```python
from build123d import *

# Parameters (mm, degrees)
BOSS_EXTRUDE1_DEPTH = 36.5
CUT_EXTRUDE1_DEPTH  = 119.232821162
SKETCH3_W           = 12
SKETCH3_H           = 22
CUT_EXTRUDE4_DEPTH  = 7
SKETCH7_R           = 1.5
CUT_EXTRUDE10_DEPTH = 8


with BuildPart() as part:
    # Sketch1 → Boss-Extrude1 (new, symmetric)
    with BuildSketch(Plane.XY):
        Polygon((-55, 0), (55, 0), (55, 15), (29.503066419, 15), (20, 75), (-20, 75), (-29.503066419, 15), (-55, 15), align=None)
    extrude(amount=BOSS_EXTRUDE1_DEPTH, both=True)

    # Sketch2 → Cut-Extrude1 (cut, through all)
    with BuildSketch(Plane.XY.offset(36.5)):
        Polygon((-22.820796589, 15), (22.820796589, 15), (25.196563194, 0), (-25.196563194, 0), align=None)
        Polygon((-21.775459283, 21.6), (21.775459283, 21.6), (14.363067476, 68.4), (-14.363067476, 68.4), align=None)
    extrude(amount=-CUT_EXTRUDE1_DEPTH, mode=Mode.SUBTRACT)

    # Sketch3 → Cut-Extrude4 (cut)
    with BuildSketch(Plane(origin=(0, 75, 0), x_dir=(1, 0, 0), z_dir=(0, 1, 0))):
        Rectangle(SKETCH3_W, SKETCH3_H)
    extrude(amount=-CUT_EXTRUDE4_DEPTH, mode=Mode.SUBTRACT)

    # Sketch7 → Cut-Extrude10 (cut)
    with BuildSketch(Plane(origin=(0, 75, 0), x_dir=(1, 0, 0), z_dir=(0, 1, 0))):
        with Locations(Location((0, 14, 0), (0, 0, 270))):
            Circle(SKETCH7_R)
        with Locations(Location((0.102187059, -13.999627059, 0), (0, 0, 270))):
            Circle(SKETCH7_R)
    extrude(amount=-CUT_EXTRUDE10_DEPTH, mode=Mode.SUBTRACT)


solid = part.part
```
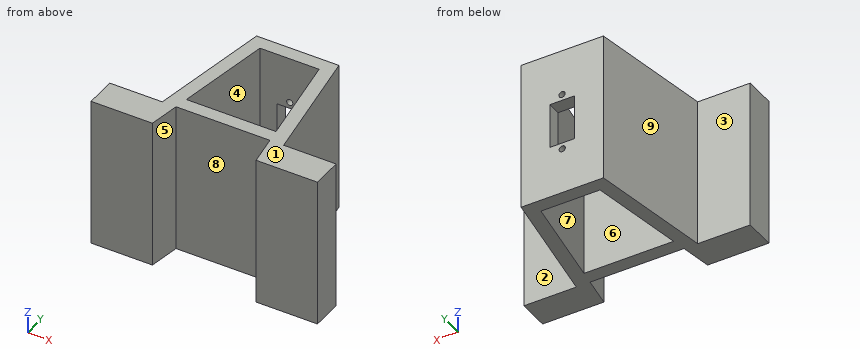
Input: part model. Units: mm. Frame: model coordinates. Face numbers are marked on the shaded views. A direction names the side the tool comes from. Coordinates: 2 decimals unless noted, no trailing zeros. Write each loop counter-clockwise with the first axis right and the second up, starting at its lowest first coordinate (ties: lowest second). Pieces come first, ordered by that corner, then holes. Notation, with made-up numbers: (20.5, -11) -> (73.5, -11) arc R6 ccw to (73.5, -1) -> close; hole circle Ø9 at (81.5, -17.75). An arc over 180 degrees is marked (long way). Write each question's results on one line, items separated by ' | '.
Item 1: Material intervals for probe 1 along Y at (x, z) = (7, -12); probe 2 along X at (y, z) = (43, 22.5); probe 3 along X at (y, z) = (47, 14), sorted ascending.
Conclusion:
probe 1: y = 15 to 21.6, 68.4 to 75 | probe 2: x = -25.07 to -18.39, 18.39 to 25.07 | probe 3: x = -24.43 to -17.75, 17.75 to 24.43
Item 2: Section query C-C on y = 66. Return loops of the section in (x, z).
Conclusion:
outline: (-21.43, -36.5) -> (-14.74, -36.5) -> (-14.74, 36.5) -> (-21.43, 36.5) -> close; (14.74, -36.5) -> (21.43, -36.5) -> (21.43, 36.5) -> (14.74, 36.5) -> close
Item 3: Set-up query: the marked faces 1, 2, 3, 4 and 5. Return all of +Z, -Z, +X, -X, +Y, -Y with unobstructed straight access to the full face (end or side cutting, diameter ignored); none if empty.
Conclusion:
face 1: +Z, +X, -X, +Y, -Y | face 2: +Z, -Z, +X, +Y | face 3: +Z, -Z, -X, +Y | face 4: +Z, -Z | face 5: +Z, -Z, -Y
Item 4: Section query B-B on z = -26. Return loops of the section in (x, y).
Conclusion:
outline: (-55, 0) -> (-25.2, 0) -> (-22.82, 15) -> (22.82, 15) -> (25.2, 0) -> (55, 0) -> (55, 15) -> (29.5, 15) -> (20, 75) -> (-20, 75) -> (-29.5, 15) -> (-55, 15) -> close; hole (-21.78, 21.6) -> (21.78, 21.6) -> (14.36, 68.4) -> (-14.36, 68.4) -> close
Item 5: Mould query, pull axis Y, two halves, no side actions, for the marked faces 6, 7, 8 and 9. Classes: +Y half, -Y half, draft (parallel to the pull), parting line (faces both ways), or undercut.
Conclusion:
face 6: undercut | face 7: undercut | face 8: -Y half | face 9: +Y half
Item 6: Pin query (flat end, axial travel): pin 1 Ø3 at (y, z) = (38.5, 12) entering from +X; pin 2 Ø12.5 at (x, z) = (-44, 0) entering from +Y; pin 3 Ø1.8 at (x, z) = (0.1, 14) entering from -Y. Return the tip coordinate at first contact, or that it passes through.
Conclusion:
pin 1: stops at x = 26.02 | pin 2: stops at y = 15 | pin 3: stops at y = 15
Item 7: Section query A-A on x = 3. Return loops of the section in (y, z).
Conclusion:
outline: (15, -36.5) -> (21.6, -36.5) -> (21.6, 36.5) -> (15, 36.5) -> close; (68.4, -36.5) -> (75, -36.5) -> (75, -11) -> (68.4, -11) -> close; (68.4, 11) -> (75, 11) -> (75, 36.5) -> (68.4, 36.5) -> close
Item 8: Section query D-D on z = -14. Return loops of the section in (x, y), plus the area to 3 significant figures.
Conclusion:
outline: (-55, 0) -> (-25.2, 0) -> (-22.82, 15) -> (22.82, 15) -> (25.2, 0) -> (55, 0) -> (55, 15) -> (29.5, 15) -> (20, 75) -> (1.5, 75) -> (1.5, 68.4) -> (14.36, 68.4) -> (21.78, 21.6) -> (-21.78, 21.6) -> (-14.36, 68.4) -> (-1.5, 68.4) -> (-1.5, 75) -> (-20, 75) -> (-29.5, 15) -> (-55, 15) -> close | area: 2,190 mm^2
